```python
from build123d import *

# Parameters (mm, degrees)
SKETCH024_W     = 9
SKETCH024_H     = 11
PAD009_DEPTH    = 12
POCKET006_DEPTH = 8.701
POCKET007_DEPTH = 8
SKETCH034_W     = 5.8
SKETCH034_H     = 3.2
POCKET008_DEPTH = 12.65
SKETCH035_W     = 3.4
SKETCH035_H     = 0.3
POCKET009_DEPTH = 9.15
SKETCH036_W     = 3.4
SKETCH036_H     = 0.3
POCKET010_DEPTH = 4.2
SKETCH037_W     = 4.6
SKETCH037_H     = 0.3
POCKET011_DEPTH = 4
SKETCH038_W     = 2
SKETCH038_H     = 1
POCKET012_DEPTH = 6.15


with BuildPart() as part:
    # Sketch024 → Pad009 (new body)
    with BuildSketch(Plane.YZ.offset(-13.5)):
        with Locations((0, 6)):
            Rectangle(SKETCH024_W, SKETCH024_H)
    extrude(amount=PAD009_DEPTH)

    # Sketch025 → Pocket006 (cut, through all)
    with BuildSketch(Plane.YZ.offset(-10.2)):
        with BuildLine():
            Line((-5, 7), (-4.2, 7))
            ThreePointArc((4.2, 7), (0, 11.2), (-4.2, 7))
            Line((4.2, 7), (5, 7))
            Line((5, 12), (5, 7))
            Line((-5, 12), (5, 12))
            Line((-5, 7), (-5, 12))
        make_face()
    extrude(amount=POCKET006_DEPTH, mode=Mode.SUBTRACT)

    # Sketch031 → Groove (revolve, cut)
    with BuildSketch(Plane.XZ):
        Polygon((-3, 8.6), (-3, 8), (0, 8), (0, 7), (-14, 7), (-14, 10.2), (-4, 10.2), (-4, 8.6), align=None)
    revolve(axis=Axis((-14, 0, 7), (-1, 0, 0)), mode=Mode.SUBTRACT)

    # Sketch032 → Pocket007 (cut)
    with BuildSketch(Plane.YZ.offset(-1.5)):
        Polygon((-2.9, 4.4), (2.9, 4.4), (2.9, 1.8), (3.4, 1.8), (3.4, 1.5), (-3.4, 1.5), (-3.4, 1.8), (-2.9, 1.8), align=None)
    extrude(amount=-POCKET007_DEPTH, mode=Mode.SUBTRACT)

    # Sketch034 → Pocket008 (cut)
    with BuildSketch(Plane.YZ):
        with Locations((0, 3.1)):
            Rectangle(SKETCH034_W, SKETCH034_H)
    extrude(amount=-POCKET008_DEPTH, mode=Mode.SUBTRACT)

    # Sketch035 → Pocket009 (cut)
    with BuildSketch(Plane.YZ):
        with Locations((-1.7, 4.55)):
            Rectangle(SKETCH035_W, SKETCH035_H)
    extrude(amount=-POCKET009_DEPTH, mode=Mode.SUBTRACT)

    # Sketch036 → Pocket010 (cut)
    with BuildSketch(Plane.YZ):
        with Locations((1.7, 4.55)):
            Rectangle(SKETCH036_W, SKETCH036_H)
    extrude(amount=-POCKET010_DEPTH, mode=Mode.SUBTRACT)

    # Sketch037 → Pocket011 (cut)
    with BuildSketch(Plane.YZ):
        with Locations((-2.3, 4.55)):
            Rectangle(SKETCH037_W, SKETCH037_H)
    extrude(amount=-POCKET011_DEPTH, mode=Mode.SUBTRACT)

    # Sketch038 → Pocket012 (cut)
    with BuildSketch(Plane.YZ):
        with Locations((0, 1)):
            Rectangle(SKETCH038_W, SKETCH038_H)
    extrude(amount=-POCKET012_DEPTH, mode=Mode.SUBTRACT)


with BuildPart() as part_1:
    # Body009 placement: moved
    add(part.part.moved(Location((0, 0, -0.5))))


solid = part_1.part
```
The model under review builds one solid part; all positions refer to its coordinate system, in mm. A direction names the side the tool comes from. Round coordinates to 2 decimals unless told otherwise and drop trailing zeros. Loops run counter-clockwise (first coordinate to the right, second up) from the corner with the lowest first, then second, coordinate; pieces in that order, holes last. Notation, with made-up numbers: (-28.5, -25) - (4.5, -25) arc R23 ccw to (4.5, 9) - close; hole circle Ø6 at (35.5, 66). An arc over 180 degrees is marked (long way). Write each question's results on one line, items separated by ' | '. Start each with the question number.
Q1. Take a section at A-A on y = 0. Give the boundary of the cut face in (x, z), plus the area to 3 significant figures.
Q2. Take a section at C-C on y = -2. Give the boundary of the cut face in (x, z).
Q3. Wall thickness on line 1 along Y through (x, z) = (-5, 2.75); line 2 along Z through (x, y) = (-7.5, 0); line 3 along Z through (x, y) = (-2.5, 0): over which ranges is each line inside the solid? List them lowest first. Write a range as [from, to].
Q4. Tool access review of faces 4 (the flat face through (-4, -1, 8)), 5 (the flat face through (-6.15, 0, 0.5)), 6 (the flat face through (-4.4, -3.2, 3.9)): name each direction out of +Z, -Z, +X, -X, +Y, -Y from which nothing blocks a thin tool from reaching the whole face with its end or side.
Q5. Draft analysis for pull direction Z (two halves, no side actions). For faces 1 (the flat face through (-12, 0, 11)), 2 (the flat face through (-1.5, 1, 5)), 3 (the flat face through (-12.65, 0, 2)), state which applies: pulls with the +Z half, pulls with the -Z half, needs draft (parallel to the pull), parting line crosses it, or undercut.
Q6. Take a section at B-B on z = 7. Give the boundary of the cut face in (x, y).
Q7. Take a section at D-D on x = -11.5. Give the boundary of the cut face in (y, z), plus the area to 3 significant figures.
Data:
1) outline: (-13.5, 0) - (-6.15, 0) - (-6.15, 1) - (-12.65, 1) - (-12.65, 3.3) - (-13.5, 3.3) - close; (-13.5, 9.7) - (-4, 9.7) - (-4, 8.1) - (-3, 8.1) - (-3, 7.5) - (-1.5, 7.5) - (-1.5, 10.7) - (-10.2, 10.7) - (-10.2, 11) - (-13.5, 11) - close; (-4, 4.2) - (-1.5, 4.2) - (-1.5, 5.5) - (-3, 5.5) - (-3, 4.9) - (-4, 4.9) - close | area: 29.8 mm²
2) outline: (-13.5, 0) - (-1.5, 0) - (-1.5, 1) - (-12.65, 1) - (-12.65, 4) - (-13.5, 4) - close; (-13.5, 9) - (-4, 9) - (-4, 4.2) - (-1.5, 4.2) - (-1.5, 10.19) - (-10.2, 10.19) - (-10.2, 11) - (-13.5, 11) - close
3) line 1: y = [-4.5, -2.9], [2.9, 4.5] | line 2: z = [0, 1], [9.7, 10.7] | line 3: z = [4.2, 5.5], [7.5, 10.7]
4) face 4: -X | face 5: -Z, +X | face 6: +X
5) face 1: pulls with the +Z half | face 2: needs draft | face 3: undercut
6) outline: (-13.5, -4.5) - (-10.2, -4.5) - (-10.2, -4.17) - (-1.5, -4.17) - (-1.5, -0.87) - (-3, -0.87) - (-3, -1.52) - (-4, -1.52) - (-4, -3.16) - (-13.5, -3.16) - close; (-13.5, 3.16) - (-4, 3.16) - (-4, 1.52) - (-3, 1.52) - (-3, 0.87) - (-1.5, 0.87) - (-1.5, 4.17) - (-10.2, 4.17) - (-10.2, 4.5) - (-13.5, 4.5) - close
7) outline: (-4.5, 0) - (4.5, 0) - (4.5, 11) - (-4.5, 11) - close; hole (-2.9, 1) - (2.9, 1) - (2.9, 4.2) - (2.22, 4.2) arc R3.2 ccw (long way) to (-2.22, 4.2) - (-2.9, 4.2) - close | area: 51.0 mm²
